For this review, take the finished solid that the model builds, in its own axes (mm). Face numbers are marked on the shaded views. A direction names the side the tool comes from. Give positions to 0.01 mm unless a question says otherwise; leave off trailing zeros. Write each loop counter-clockwise with the first axis right and the second up, starting at its lowest first coordinate (ties: lowest second). Pieces come first, ordered by that corner, then holes.
1) We need section B-B on z = -6.5. Give the boundary of the cut face in (x, y), and give its area (3 significant figures).
2) For P1, Ø12, axis at y = 99, z = -0.5, coming from the -X side; P2, Ø4, axis at x = -13, z = -6.5, coming from the +Y side; P3, Ø12, axis at x = 22, z = -4.5, coming from the +Y side; P4, Ø4, axis at y = 61, z = -6, coming from the +X side, all flat-tipped, find the tip position at first contact; note any pin that passes through.
3) Machinability: for the marked faces 1, 2 and 3, which of the approach directions +Z, -Z, +X, -X, +Y, -Y give a long, thin tool a straight path to every point of the face, cutting with its end or side? Answer none if there is none.
4) Wall thickness on line 1 along X through (y, z) = (143.25, -6.5); line 2 along Z through (x, y) = (-13, 140); line 3 along X through (y, z) = (140, -8.25): over which ranges is each line inside the solid? List them lowest first.
5) We need section A-A on x = -25. Give the boundary of the cut face in (y, z).
6) We need section C-C on x = -13. Give the boundary of the cut face in (y, z).
7) We need section D-D on y = 112. Give the boundary of the cut face in (x, z).
from build123d import *

# Parameters (mm, degrees)
ESBO_O1_W                = 60
ESBO_O1_H                = 25
RESSALTO_EXTRUS_O1_DEPTH = 10
ESBO_O7_W                = 38
ESBO_O7_H                = 25
RESSALTO_EXTRUS_O3_DEPTH = 140
ESBO_O8_R                = 2.5
CORTE_EXTRUS_O4_DEPTH    = 20
CORTE_EXTRUS_O5_DEPTH    = 20


with BuildPart() as part:
    # Esboço1 → Ressalto-extrusão1 (new body)
    with BuildSketch(Plane(origin=(0, 0, 0), x_dir=(1, 0, 0), z_dir=(0, 1, 0))):
        Rectangle(ESBO_O1_W, ESBO_O1_H)
    extrude(amount=RESSALTO_EXTRUS_O1_DEPTH)

    # Esboço7 → Ressalto-extrusão3 (add)
    with BuildSketch(Plane(origin=(0, 10, 0), x_dir=(1, 0, 0), z_dir=(0, 1, 0))):
        Rectangle(ESBO_O7_W, ESBO_O7_H)
    extrude(amount=RESSALTO_EXTRUS_O3_DEPTH)

    # Esboço8 → Corte-extrusão4 (cut)
    with BuildSketch(Plane(origin=(0, 150, 0), x_dir=(1, 0, 0), z_dir=(0, 1, 0))):
        with Locations((-13, 6.5)):
            Circle(ESBO_O8_R)
        with Locations((15, 6.5)):
            Circle(ESBO_O8_R)
    extrude(amount=-CORTE_EXTRUS_O4_DEPTH, mode=Mode.SUBTRACT)

    # Esboço9 → Corte-extrusão5 (cut)
    with BuildSketch(Plane(origin=(0, 10, 0), x_dir=(1, 0, 0), z_dir=(0, 1, 0))):
        with BuildLine():
            Line((-28.2, -4.5), (-28.2, -0.5))
            ThreePointArc((-28.2, -0.5), (-25, 2.7), (-21.8, -0.5))
            Line((-21.8, -0.5), (-21.8, -4.5))
            ThreePointArc((-21.8, -4.5), (-25, -7.7), (-28.2, -4.5))
        make_face()
        with BuildLine():
            Line((21.8, -4.5), (21.8, -0.5))
            ThreePointArc((21.8, -0.5), (25, 2.7), (28.2, -0.5))
            Line((28.2, -0.5), (28.2, -4.5))
            ThreePointArc((28.2, -4.5), (25, -7.7), (21.8, -4.5))
        make_face()
    extrude(amount=-CORTE_EXTRUS_O5_DEPTH, mode=Mode.SUBTRACT)


solid = part.part
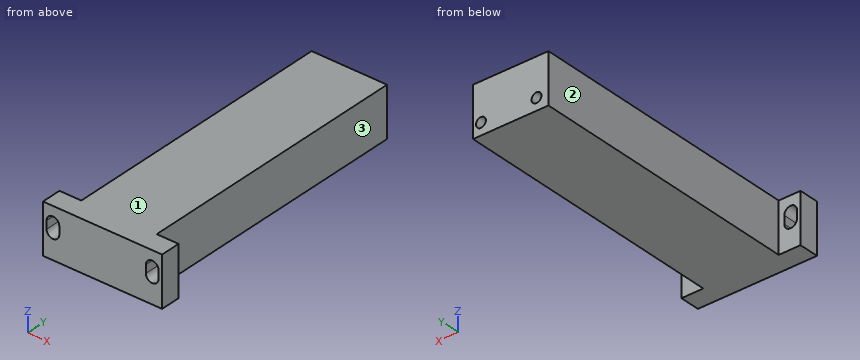
Results list:
1. outline: (-30, 0) - (30, 0) - (30, 10) - (19, 10) - (19, 150) - (17.5, 150) - (17.5, 130) - (12.5, 130) - (12.5, 150) - (-10.5, 150) - (-10.5, 130) - (-15.5, 130) - (-15.5, 150) - (-19, 150) - (-19, 10) - (-30, 10) - close
1. area: 5,720 mm2
2. P1: stops at x = -19
2. P2: stops at y = 130
2. P3: stops at y = 150
2. P4: stops at x = 19
3. face 1: +Z, +X, -X, +Y, -Y
3. face 2: +Z, -Z, -X, +Y
3. face 3: +Z, -Z, +X, +Y
4. line 1: x = -19 to -15.5, -10.5 to 12.5, 17.5 to 19
4. line 2: z = -12.5 to -9, -4 to 12.5
4. line 3: x = -19 to -14.79, -11.21 to 13.21, 16.79 to 19
5. outline: (0, -12.5) - (10, -12.5) - (10, -2.7) - (0, -2.7) - close; (0, 7.7) - (10, 7.7) - (10, 12.5) - (0, 12.5) - close
6. outline: (0, -12.5) - (150, -12.5) - (150, -9) - (130, -9) - (130, -4) - (150, -4) - (150, 12.5) - (0, 12.5) - close
7. outline: (-19, -12.5) - (19, -12.5) - (19, 12.5) - (-19, 12.5) - close
